Input: part model. Units: mm. Frame: model coordinates. A direction names the side the tool comes from. Round coordinates to 2 decimals unless told otherwise and drop trailing zeros. Order: outer loops, then holes, each group sorted by start corner. A loop starts at its lowest first (then second) coordinate and runs counter-clockwise, first axis right, second up. Notation, with made-up numbers: (-15.5, -28) - (39.5, -28) arc R20 cw to (39.5, 4) - close; hole circle Ø10 at (-33.5, -15.75). An arc over 180 degrees is marked (long way). One line per item, written item: value. Start each with the question number.
from build123d import *

# Parameters (mm, degrees)
F2_R     = 67.2650557496
F2_R_2   = 5.08
F2_R_3   = 20.066
F3_DEPTH = 7
F1_R     = 5.08
F1_R_2   = 2.54
F4_DEPTH = 3.5
F5_SIZE  = 1.27


with BuildPart() as f3:
    # F2 (on Top) → F3 (new body)
    with BuildSketch(Plane.XY):
        Circle(F2_R)
        with Locations((-37.846, -36.957)):
            Circle(F2_R_2, mode=Mode.SUBTRACT)
        with Locations((37.846, -36.957)):
            Circle(F2_R_2, mode=Mode.SUBTRACT)
        with Locations((-37.846, 30.9118)):
            Circle(F2_R_2, mode=Mode.SUBTRACT)
        Circle(F2_R_3, mode=Mode.SUBTRACT)
        with Locations((37.846, 30.9118)):
            Circle(F2_R_2, mode=Mode.SUBTRACT)
    extrude(amount=F3_DEPTH)

    # F1 (on Top) → F4 (join)
    with BuildSketch(Plane.XY):
        with Locations((-37.846, 30.9118)):
            Circle(F1_R)
        with Locations((-37.846, 30.9118)):
            Circle(F1_R_2, mode=Mode.SUBTRACT)
        with Locations((37.846, 30.9118)):
            Circle(F1_R)
        with Locations((37.846, 30.9118)):
            Circle(F1_R_2, mode=Mode.SUBTRACT)
        with Locations((37.846, -36.957)):
            Circle(F1_R)
        with Locations((37.846, -36.957)):
            Circle(F1_R_2, mode=Mode.SUBTRACT)
        with Locations((-37.846, -36.957)):
            Circle(F1_R)
        with Locations((-37.846, -36.957)):
            Circle(F1_R_2, mode=Mode.SUBTRACT)
    extrude(amount=F4_DEPTH)

    # F5
    f5_edges = [f3.edges().sort_by_distance(p)[0] for p in [
        (-67.265056, 0, 0),
        (-67.265056, 0, 7),
    ]]
    chamfer(f5_edges, length=F5_SIZE)


solid = f3.part
Item 1: Reachability of faces 5 (the face through (-36.481, 33.054, 1.726)), 6 (the face through (40.577, -32.674, 5.226)) from +Z, -Z, +X, -X, +Y, -Y: full face, straight path, thin tool, end or side. Return the list, or none.
Item 2: First-contact query: pin 1 Ø13 at (x, y) = (-37.85, 30.91) entering from +Z; pin 2 Ø3 at (x, z) = (5.5, 3) entering from -Y; pin 3 Ø4 at (y, z) = (36.5, 5.5) entering from -X; pin 4 Ø5 at (x, y) = (39.5, -38) entering from +Z. Flat tips, straight axial feed; report the tip coordinate or a pass-through.
Item 3: Pull-direction query (Y, two-part tool) for faces 1 (the face through (14, 16, 0)), 2 (the face through (40, 29, 3.5)), 3 (the face through (39.211, 33.054, 1.726)), 4 (the face through (-14.582, -65.666, 3.469)); classes: released by +Y, released by -Y, zero draft, split by the parting line, or undercut.
Item 4: Section query A-A on y = 0. Return loops of the section in (x, z), and give its area (3 significant figures).
Item 5: Line query: L1, parallel to Y at x = -34.5, z = 6.5; L2, parallel to X at y = -38.5, z = 5; L3, parallel to X at y = 1.5, z = 4.75. Output: solid intervals per line, ascending.
Geometry results:
1. face 5: +Z, -Z
1. face 6: +Z
2. pin 1: stops at z = 7
2. pin 2: stops at y = -67.15
2. pin 3: stops at x = -57.74
2. pin 4: stops at z = 3.5
3. face 1: zero draft
3. face 2: undercut
3. face 3: undercut
3. face 4: split by the parting line
4. outline: (-67.27, 1.27) - (-66, 0) - (-20.07, 0) - (-20.07, 7) - (-66, 7) - (-67.27, 5.73) - close; (20.07, 0) - (66, 0) - (67.27, 1.27) - (67.27, 5.73) - (66, 7) - (20.07, 7) - close
4. area: 658 mm^2
5. L1: y = -56.84 to -40.78, -33.13 to 27.09, 34.73 to 56.84
5. L2: x = -55.16 to -42.69, -33.01 to 33.01, 42.69 to 55.16
5. L3: x = -67.25 to -20.01, 20.01 to 67.25
